Answer from the drawing. Dimensions are ordinates in mm from the lowest x, y and z of the part. A direction names the side the tool comes from. Coordinates: 2 decimals unless noted, no trailing zeros. Write each loop counter-clockwise with the first axis right and the second up, starting at its lowest first coordinate (ties: lowest second). Pieces come first, ordered by that corner, then holes. Notation, with made-up numbers: (71.5, -27) -> (80.5, -27) arc R22 cw to (80.5, -12) -> close; hole circle Ø2 at (69, -14.5). An arc over 180 degrees is marked (long way). Answer as a JSON object with one key per item and string values. Group by question number.
(1) Find section C-C (y = 15). Give the vertices of the cut face in (x, z).
(2) Find section A-A (z = 51). Give the vertices of the cut face in (x, y), then the cut area to 3 significant figures.
(3) Which of the six approach directions +Z, -Z, +X, -X, +Y, -Y give full straight-line access (tool end or side, diameter ignored) to the marked faces 1 and 2?
(4) Find section B-B (x = 127.5). Give the vertices of the cut face in (y, z).
(5) For a pull along Y with two mould halves and no side action, classify the marked faces 3, 4, 5 and 6 as +Y half, -Y half, draft (parallel to the pull), parting line (faces both ways), or undercut.
(6) Straight lines are drawn through the part: L1, parallel to Y at x = 147.5, z = 23; L2, parallel to X at y = 13.5, z = 89.5; L3, parallel to X at y = 80, z = 87.5. For each, find the intervals that lie inside material, in ascending order.
(7) A flat-ended cylindrical pin translates along its axis: P1, Ø3, axis at x = 130, y = 60.5, coming from the +Z side. Find the tip coordinate at first contact, or state that the pin passes through.
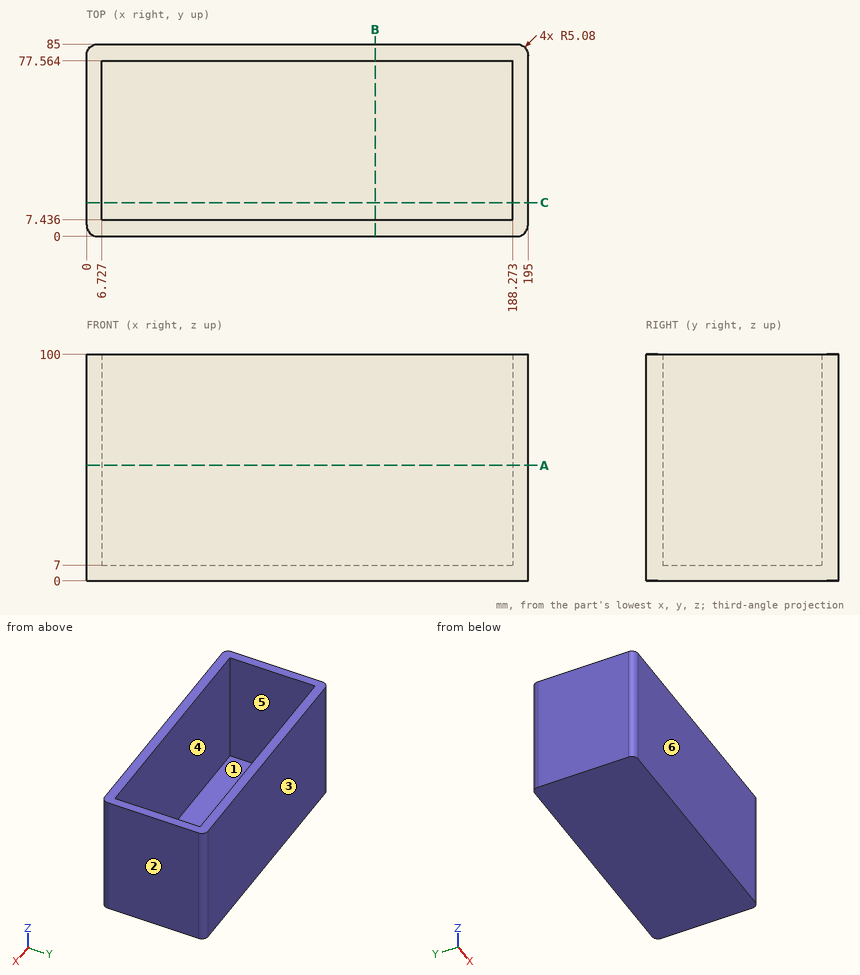
Results below:
{
 "1": {"outline": "(0, 0) -> (195, 0) -> (195, 100) -> (188.27, 100) -> (188.27, 7) -> (6.73, 7) -> (6.73, 100) -> (0, 100) -> close"},
 "2": {"outline": "(0, 5.08) arc R5.08 ccw to (5.08, 0) -> (189.92, 0) arc R5.08 ccw to (195, 5.08) -> (195, 79.92) arc R5.08 ccw to (189.92, 85) -> (5.08, 85) arc R5.08 ccw to (0, 79.92) -> close; hole (6.73, 7.44) -> (188.27, 7.44) -> (188.27, 77.56) -> (6.73, 77.56) -> close", "area": "3,820 mm2"},
 "3": {"face 1": "+Z", "face 2": "+Z, -Z, +X, +Y, -Y"},
 "4": {"outline": "(0, 0) -> (85, 0) -> (85, 100) -> (77.56, 100) -> (77.56, 7) -> (7.44, 7) -> (7.44, 100) -> (0, 100) -> close"},
 "5": {"face 3": "+Y half", "face 4": "undercut", "face 5": "undercut", "face 6": "-Y half"},
 "6": {"L1": "y = 0 to 7.44, 77.56 to 85", "L2": "x = 0 to 6.73, 188.27 to 195", "L3": "x = 0 to 195"},
 "7": {"P1": "stops at z = 7"}
}
